from build123d import *

# Parameters (mm, degrees)
SKETCH3_W          = 10.5
SKETCH3_H          = 7.752761779
CUT_EXTRUDE1_DEPTH = 83


with BuildPart() as part:
    # Sketch1 → Loft1 section 0
    with BuildSketch(Plane(origin=(0, 0, 0), x_dir=(1, 0, 0), z_dir=(0, 1, 0))):
        with BuildLine():
            Line((-11.888349515, -12.616504854), (11.611650485, -12.616504854))
            Line((11.611650485, -12.616504854), (11.611650485, 0.383495146))
            Line((11.611650485, 0.383495146), (-11.888349515, 0.383495146))
            Line((-11.888349515, 0.383495146), (-11.888349515, -12.616504854))
        make_face()
    # Sketch2 → Loft1 section 1
    with BuildSketch(Plane(origin=(0, 86, 0), x_dir=(1, 0, 0), z_dir=(0, 1, 0))):
        with BuildLine():
            Line((-10.903349515, -12.616504854), (-10.903349515, 0.383495146))
            Line((-10.903349515, 0.383495146), (10.626650485, 0.383495146))
            Line((10.626650485, 0.383495146), (10.626650485, -12.616504854))
            Line((10.626650485, -12.616504854), (-10.903349515, -12.616504854))
        make_face()
    loft()

    # Sketch3 → Cut-Extrude1 (cut)
    with BuildSketch(Plane(origin=(0, 86, 0), x_dir=(1, 0, 0), z_dir=(0, 1, 0))):
        with Locations((-1.638349515, -3.492885744)):
            Rectangle(SKETCH3_W, SKETCH3_H)
    extrude(amount=-CUT_EXTRUDE1_DEPTH, mode=Mode.SUBTRACT)


solid = part.part
The listing builds one solid part. Answer for the finished solid, in the listing's coordinates (mm). A direction names the side the tool comes from. Coordinates: 2 decimals unless noted, no trailing zeros. Loops run counter-clockwise (first coordinate to the right, second up) from the corner with the lowest first, then second, coordinate; pieces in that order, holes last.
1) Flat-ended cylindrical pins translate along their axes: pin 1 Ø1 at (y, z) = (18.5, 8) entering from +X; pin 2 Ø6 at (x, z) = (-0.5, 5) entering from +Y; pin 3 Ø1.5 at (y, z) = (67, 5.5) entering from +X; pin 4 Ø4 at (y, z) = (76.5, 3) entering from -X. Find the tip coordinate at first contact, or state that the pin passes through.
2) Find section B-B on z = 9.25. Write down the section's boundary in (x, y).
3) Find the intervals of material crossed by L1, parallel to Z at x = -3.25, y = 68; L2, parallel to Y at x = -3.5, z = 0.75; L3, parallel to X at y = 26, z = 4.5, in increasing order.
4) Find section A-A on z = 1.75. Write down the section's boundary in (x, y).
5) Determine the mould class of faces 1 (the face through (-2, 45, 7.369)), 2 (the face through (1, 86, 9)) for opening direction X: pulls with the +X half, pulls with the -X half, needs draft (parallel to the pull), parting line crosses it, or undercut.
6) A tool of negligible diameter and unlimited length cuts with its end or side. For faces 3 (the face through (-2, 3, 3)), 4 (the face through (0, 0, 6)), from which of +Z, -Z, +X, -X, +Y, -Y can it reach the whole face along a straight path? Write none if from no direction.
Values:
1. pin 1: stops at x = 11.41
1. pin 2: stops at y = 86
1. pin 3: stops at x = 10.85
1. pin 4: stops at x = -11.04
2. outline: (-11.89, 0) - (11.61, 0) - (10.63, 86) - (-10.9, 86) - close
3. L1: z = 7.37 to 12.62
3. L2: y = 0 to 3
3. L3: x = -11.59 to -6.89, 3.61 to 11.31
4. outline: (-11.89, 0) - (11.61, 0) - (10.63, 86) - (3.61, 86) - (3.61, 3) - (-6.89, 3) - (-6.89, 86) - (-10.9, 86) - close
5. face 1: undercut
5. face 2: needs draft
6. face 3: -Z, +Y
6. face 4: +Z, -Z, +X, -X, -Y
